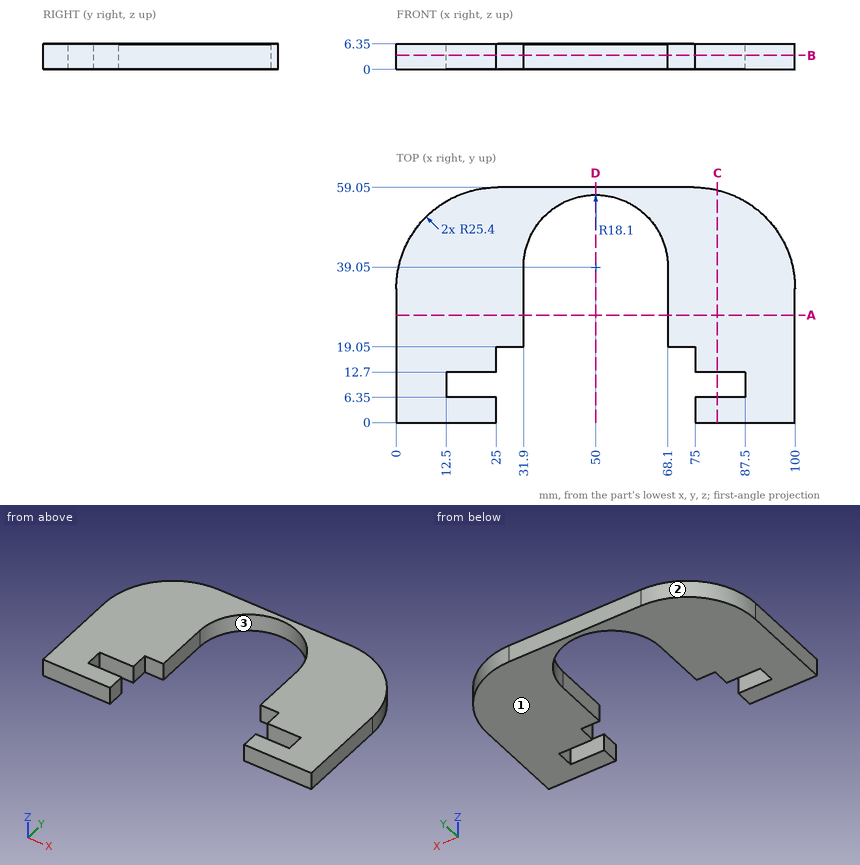
The figure shows three views and two pictorial views of one solid part (mm, origin at its lowest corner). Answer the questions. Round coordinates to 2 decimals unless told otherwise and drop trailing zeros. Loops run counter-clockwise (first coordinate to the right, second up) from the corner with the lowest first, then second, coordinate; pieces in that order, holes last. Notation, with made-up numbers: (69.25, -17) - (107.25, -17) arc R25 ccw to (107.25, 4) - close; hole circle Ø4 at (-26, 32). An arc over 180 degrees is marked (long way). One line per question, with ' | ' between items. Start each with the question number.
Q1. Section A-A on y = 27 is taken. Give the vertices of the cut face in (x, z), plus the area to 3 significant figures.
Q2. Section C-C on x = 80.5 is taken. Give the vertices of the cut face in (y, z).
Q3. Section B-B on z = 3.5 is taken. Give the vertices of the cut face in (x, y).
Q4. Section D-D on x = 50 is taken. Give the vertices of the cut face in (y, z), plus the area to 3 significant figures.
Q5. For a pull along X with two mould halves and no side action, classify the marked faces 1, 2 and 3 as +X half, -X half, draft (parallel to the pull), parting line (faces both ways), or undercut.
Q6. Find the intervals of material crossed by L1, parallel to X at y = 31, z = 3.25; L2, parallel to X at y = 48, z = 4.5; L3, parallel to Y at x = 29.5, z = 0.5, in increasing order.
Q7. Flat-ended cylindrical pins translate along their axes: pin 1 (1.9 mm diameter, centred on x = 29.5, z = 4.5, fed in from -Y); pin 2 (1 mm diameter, centred on x = 43, z = 3.5, fed in from -Y). Find the tip coordinate at first contact, or state that the pin passes through.
Established:
1) outline: (0, 0) - (31.9, 0) - (31.9, 6.35) - (0, 6.35) - close; (68.1, 0) - (100, 0) - (100, 6.35) - (68.1, 6.35) - close | area: 405 mm²
2) outline: (0, 0) - (6.35, 0) - (6.35, 6.35) - (0, 6.35) - close; (12.7, 0) - (58.36, 0) - (58.36, 6.35) - (12.7, 6.35) - close
3) outline: (0, 0) - (25, 0) - (25, 6.35) - (12.5, 6.35) - (12.5, 12.7) - (25, 12.7) - (25, 19.05) - (31.9, 19.05) - (31.9, 39.05) arc R18.1 cw to (68.1, 39.05) - (68.1, 19.05) - (75, 19.05) - (75, 12.7) - (87.5, 12.7) - (87.5, 6.35) - (75, 6.35) - (75, 0) - (100, 0) - (100, 33.65) arc R25.4 ccw to (74.6, 59.05) - (25.4, 59.05) arc R25.4 ccw to (0, 33.65) - close
4) outline: (57.15, 0) - (59.05, 0) - (59.05, 6.35) - (57.15, 6.35) - close | area: 12.1 mm²
5) face 1: draft | face 2: -X half | face 3: undercut
6) L1: 0 to 31.9, 68.1 to 100 | L2: 4.44 to 34.27, 65.73 to 95.56 | L3: 19.05 to 59.05
7) pin 1: y = 19.05 | pin 2: y = 55.52
